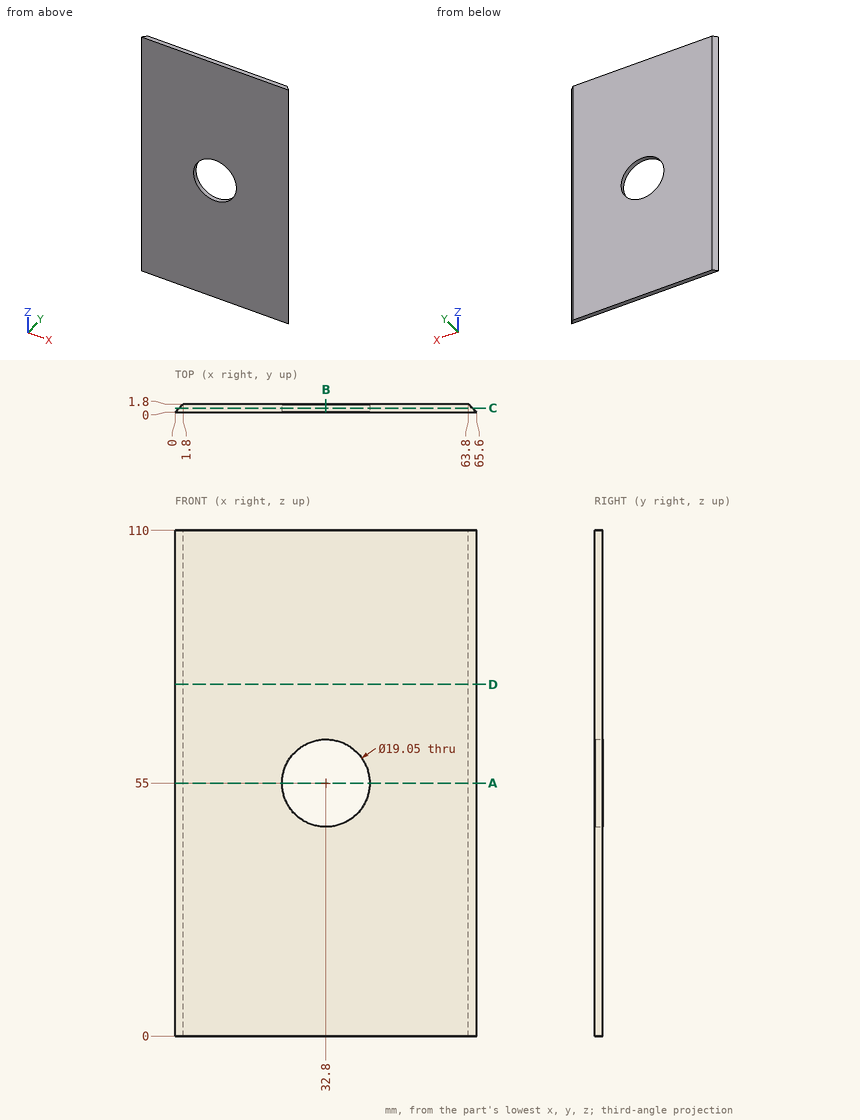
Check sheet for the drawn part. Datum: minimum x, y, z corner. Units: mm. Coordinates: 2 decimals unless noted, no trailing zeros. Order: outer loops, then holes, each group sorted by start corner. A loop starts at its lowest first (then second) coordinate and runs counter-clockwise, first axis right, second up. Notation, with made-up numbers: (-37, 33) - (-2, 33) arc R23 ccw to (-2, 71) - close; hole circle Ø7 at (54, -29.75). An arc over 180 degrees is marked (long way). Return JSON: item names as keys, results as strings.
(1) Thickness scan on line 1 along Z through (x, y) = (32.8, 1.25) (3 decimals); line 2 along X through (y, z) = (0.75, 55) (3 decimals); line 3 along X through (y, z) = (0.85, 58). Record the ranges inside material, lowest first.
Filled sheet:
{"line 1": "z = 0 to 45.475, 64.525 to 110", "line 2": "x = 0.75 to 23.275, 42.325 to 64.85", "line 3": "x = 0.85 to 23.76, 41.84 to 64.75"}
(2) Section check D-D, the plane z = 76.5. Record the cut outline in (x, y), and give its area (3 significant figures).
Filled sheet:
{"outline": "(0, 0) - (65.6, 0) - (63.8, 1.8) - (1.8, 1.8) - close", "area": "115 mm^2"}
(3) Section check B-B, the plane x = 32.8. Record the cut outline in (y, z) (3 decimals).
Filled sheet:
{"outline": "(0, 0) - (1.8, 0) - (1.8, 45.475) - (0, 45.475) - close; (0, 64.525) - (1.8, 64.525) - (1.8, 110) - (0, 110) - close"}
(4) Section check C-C, the plane y = 0.9. Record the cut outline in (x, z) (3 decimals).
Filled sheet:
{"outline": "(0.9, 0) - (64.7, 0) - (64.7, 110) - (0.9, 110) - close; hole circle Ø19.05 at (32.8, 55)"}
(5) Section check A-A, the plane z = 55. Record the cut outline in (x, y) (3 decimals).
Filled sheet:
{"outline": "(0, 0) - (23.275, 0) - (23.275, 1.8) - (1.8, 1.8) - close; (42.325, 0) - (65.6, 0) - (63.8, 1.8) - (42.325, 1.8) - close"}
